Part print with two shaded views. Sizes in mm from the minimum x, y, z corner. A direction names the side the tool comes from. Coordinates: 2 decimals unless noted, no trailing zeros. Write each loop counter-clockwise with the first axis right and the second up, starting at its lowest first coordinate (ties: lowest second). Pieces come first, ordered by that corner, then holes. Notation, with made-up numbers: (82, 71) -> (98, 71) arc R34 cw to (98, 108) -> close; hole circle Ø3 at (76, 4.25). An arc over 180 degrees is marked (long way). Write item = value, one per line. Start each with the question number.
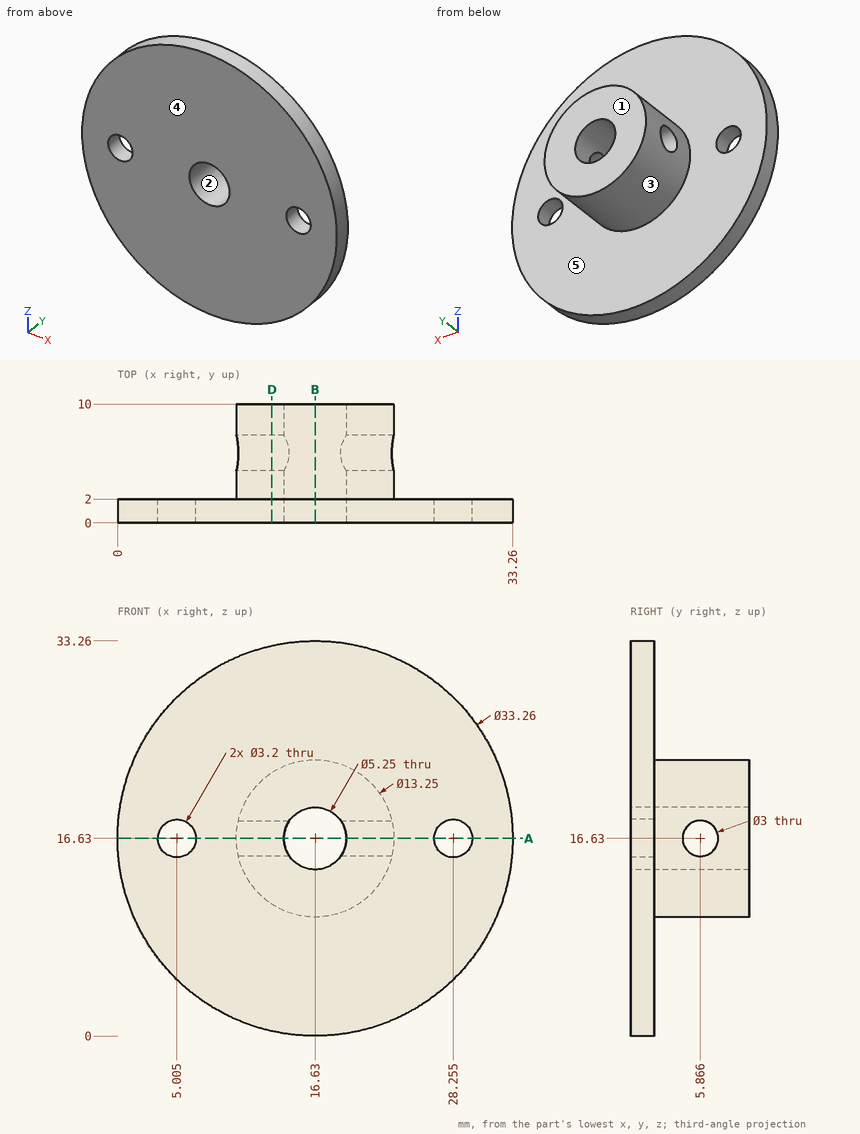
(1) 3-axis set-ups, long thin cutter, end or side, ignore diameter. For the marked faces 4 and 5: which of +Z, -Z, +X, -X, +Y, -Y reach the whole face in a straight line?
(2) Drop flat-ended pins along their axis: pin 1 Ø5 at (y, z) = (5.87, 16.63) entering from -X (3 decimals); pin 2 Ø4 at (x, z) = (29.5, 15) entering from +Y; pin 3 Ø2 at (y, z) = (1.5, 28.5) entering from +X (1 decimal); pin 4 Ø2.5 at (x, z) = (28.255, 16.63) entering from +Y. Give the stop position or say it passes through.
(3) Saw through at D-D (x = 13). Give the cut face in (y, z).
(4) Mould opens along Z. For the marked faces 1, 2 and 3 say: released by +Z, released by -Z, zero draft, split by the parting line, or undercut.
(5) Drill centre lines: line 1 along X through (y, z) = (1.4, 16.63) (1 decimal); line 2 along Y through (x, z) = (21.15, 16.63); line 3 along Y through (x, z) = (22, 10.5). Where is each one in solid material? Low to high.
(6) Saw through at A-A (z = 16.63). Give the cut face in (x, y) (1 decimal).
(7) Saw through at B-B (x = 16.63). Give the cut face in (y, z) (1 decimal), then the cut area to 3 significant figures.
Returned:
q1.face_4 = +Z, -Z, +X, -X, -Y
q1.face_5 = +Y
q2.pin_1 = 10.005
q2.pin_2 = 2
q2.pin_3 = 29.2
q2.pin_4 = through
q3.outline = (0, 0.4) -> (2, 0.4) -> (2, 11.09) -> (10, 11.09) -> (10, 22.17) -> (2, 22.17) -> (2, 32.86) -> (0, 32.86) -> close; hole circle Ø3 at (5.87, 16.63)
q4.face_1 = zero draft
q4.face_2 = undercut
q4.face_3 = split by the parting line
q5.line_1 = 0 to 3.4, 6.6 to 14, 19.3 to 26.7, 29.9 to 33.3
q5.line_2 = 0 to 4.37, 7.37 to 10
q5.line_3 = 0 to 2
q6.outline = (0, 0) -> (3.4, 0) -> (3.4, 2) -> (0, 2) -> close; (6.6, 0) -> (14, 0) -> (14, 4.4) -> (10, 4.4) -> (10, 2) -> (6.6, 2) -> close; (10, 7.4) -> (14, 7.4) -> (14, 10) -> (10, 10) -> close; (19.3, 0) -> (26.7, 0) -> (26.7, 2) -> (23.3, 2) -> (23.3, 4.4) -> (19.3, 4.4) -> close; (19.3, 7.4) -> (23.3, 7.4) -> (23.3, 10) -> (19.3, 10) -> close; (29.9, 0) -> (33.3, 0) -> (33.3, 2) -> (29.9, 2) -> close
q7.outline = (0, 0) -> (2, 0) -> (2, 10) -> (10, 10) -> (10, 14) -> (0, 14) -> close; (0, 19.3) -> (10, 19.3) -> (10, 23.3) -> (2, 23.3) -> (2, 33.3) -> (0, 33.3) -> close
q7.area = 120 mm2
